Autodesk Inventor part; units mm, degrees
ref_plane "Work Plane1" through (1.525, 0, 0) normal (0, 0, 1) x (1, 0, 0)
ref_plane "YZ Plane" through (0, 0, 0) normal (1, 0, 0) x (0, 1, 0)
ref_plane "XZ Plane" through (0, 0, 0) normal (0, 1, 0) x (-1, 0, 0)
sketch "Sketch1" plane through (0, 0, 0) normal (0, 0, 1) x (1, 0, 0)
  line L0 (0, 11.25) -> (0, 8)
  line L1 (6, 8) -> (25, 8)
  line L2 (25, 8) -> (25, 0)
  line L3 (25, 0) -> (-0.8001, 0)
  line L4 (-5.9601, 0) -> (30.16, 0)
  line L5 (-0.8001, 0) -> (-0.8001, 11.25)
  line L6 (-0.8001, 11.25) -> (0, 11.25)
  line L7 (6, 8) -> (4.773, 8)
  line L8 (4.773, 8) -> (0, 8)
  line L9 (0, -2.25) -> (0, 13.5)
  dimension "d0" = 25
  dimension "d1" = 19
  dimension "d2" = 16
  dimension "d9" = 0.8001
  dimension "d10" = 22.5
  dimension "d13" = 1.227
  dimension "d14" = 16
revolve "Body" add sketch "Sketch1" angle 360 about axis through (25, 0, 0) along (-1, 0, 0)
sketch "Sketch2" plane through (-0.8001, 0, 0) normal (-1, 0, 0) x (0, 0, 1)
  line L0 (0, 13.8564) -> (12, 6.9282)
  line L1 (12, 6.9282) -> (12, -6.9282)
  line L2 (12, -6.9282) -> (0, -13.8564)
  line L3 (0, -13.8564) -> (-12, -6.9282)
  line L4 (-12, -6.9282) -> (-12, 6.9282)
  line L5 (-12, 6.9282) -> (0, 13.8564)
  point P0 (0, 0)
  point P1 (0, 0)
  dimension "d11" = 24
extrude "Head" add sketch "Sketch2" along normal blind 9.2
sketch "Sketch4" plane through (0, 0, 0) normal (0, 0, 1) x (1, 0, 0)
  line L0 (-10.0001, 12) -> (-10.0001, 13.8564)
  line L1 (-10.0001, 13.8564) -> (-8.9283, 13.8564)
  line L2 (-8.9283, 13.8564) -> (-10.0001, 12)
  line L3 (-11.8401, 0) -> (1.0399, 0)
  line L4 (-0.8001, 13.8564) -> (-10.0001, 13.8564)
  line L5 (-10.0001, 6.9282) -> (-10.0001, 13.8564)
  dimension "d5" = 30
  dimension "d19" = 24
revolve "Chamfer1" cut sketch "Sketch4" angle 360 about axis through (-10, 0, 0) along (1, 0, 0)
thread "Thread"
chamfer "Chamfer2" distance 1.2269 distance2 1.227 1 edges at (25, -8, 0) measured on face at (25, -1.5148, -1.342)
ref_plane "Work Plane1" through (1.525, 0, 0) normal (0, 0, 1) x (1, 0, 0)
equation "\"d0\" = NLG"
equation "\"d1\" = GEL"
equation "\"d2\" = GD"
equation "\"d10\" = SD2"
equation "\"d14\" = BDM"
equation "\"d11\" = SW"
equation "\"d3\" = KOH - SD"
equation "\"d5\" = ANG1"
equation "\"d19\" = SW0"
equation "\"d15\" = GEL"
equation "\"d6\" = -0.5 * SPD + 0.5 * GD"
equation "\"NLG\" = 25"
equation "\"GD\" = NND"
equation "\"BDM\" = NND"
equation "\"KOH\" = 10"
equation "\"GEL\" = 19"
equation "\"SW\" = 24"
equation "\"SW0\" = SW"
equation "\"SPD\" = NND - 1.2269 * PTC"
equation "\"SD2\" = SDH"
equation "\"SD\" = 0.8"
equation "\"ANG1\" = 30deg"
equation "\"GAL\" = 0.61345 * PTC"
equation "\"GUL\" = 0.61345 * PTC"
equation "\"RR\" = 0.6"
equation "\"WFT\" = SD"
equation "\"GD1\" = THREADDIA - 1.2269 * PTC"
equation "\"THREADDIA\" = 16"
equation "\"SDH\" = 22.5"
equation "\"SDHG\" = GAL"
equation "\"TOA\" = 30deg"
equation "\"FAWI\" = 45deg"
equation "\"PTC\" = 2"
equation "\"NND\" = 16"
equation "\"E0\" = 1.155 * SW"
properties part number "Bolt M16x25-8.8-A PN-85/M-82105" material "Steel, Mild"
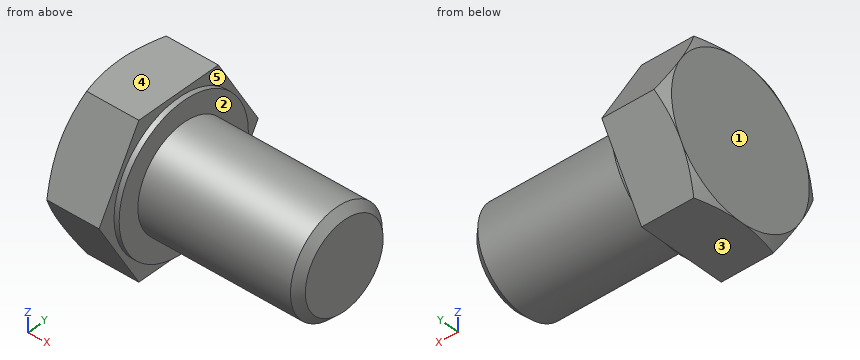
Geometry: final body of the model. Coordinates: model frame, mm. Face numbers are marked on the shaded views. A direction names the side the tool comes from. Coordinates: 2 decimals unless noted, no trailing zeros. Loops run counter-clockwise (first coordinate to the right, second up) from the corner with the lowest first, then second, coordinate; pieces in that order, holes last. Notation, with made-up numbers: (46.25, -21) -> (62.25, -21) arc R33 cw to (62.25, 12) -> close; hole circle Ø5 at (13.5, 81). An arc over 180 degrees is marked (long way). Use a Markdown table: item, result. Add a question column.
(1) Mould query, pull axis X, two halves, no side actions, for the marked faces 1, 2 and 3. Classes: pulls with the +X half, pulls with the -X half, needs draft (parallel to the pull), parting line crosses it, or undercut.
(2) Section query A-A, the plane x = 18.5. Return loops of the section in (y, z).
(3) Access query for the marked faces 4 and 5. Directions: +Z, -Z, +X, -X, +Y, -Y. A direction counts if a zero-diameter tool reaches every point of the face in a straight line with its end or side. Return the directions, or none.
(4) Line query: line 1 along Y through (x, z) = (6, 0.25); line 2 along X through (y, z) = (-7.5, 6.5); line 3 along Z through (x, y) = (15.5, 3). Output: solid intervals per line, ascending.
(5) Pin query (flat end, axial travel): pin 1 Ø12 at (x, y) = (17.5, 3.5) entering from +Z; pin 2 Ø6 at (x, z) = (16, -6) entering from +Y; pin 3 Ø6 at (y, z) = (10, -4.5) entering from +X; pin 4 Ø1 at (y, z) = (10, 8.5) entering from -X. Return the tip coordinate at first contact, or that it passes through.
Answer:
| question | item | result |
|---|---|---|
| 1 | face 1 | pulls with the -X half |
| 1 | face 2 | pulls with the +X half |
| 1 | face 3 | needs draft |
| 2 | outline | circle Ø16 at (0, 0) |
| 3 | face 4 | +Z, +X, -X, +Y, -Y |
| 3 | face 5 | +X |
| 4 | line 1 | y = -8 to 8 |
| 4 | line 2 | x = -10 to 0 |
| 4 | line 3 | z = -7.42 to 7.42 |
| 5 | pin 1 | stops at z = 8 |
| 5 | pin 2 | stops at y = 7.42 |
| 5 | pin 3 | stops at x = 23.81 |
| 5 | pin 4 | passes through |
